Verification items for the finished model (mm, model axes). A direction names the side the tool comes from. Round coordinates to 2 decimals unless told otherwise and drop trailing zeros. Write each loop counter-clockwise with the first axis right and the second up, starting at its lowest first coordinate (ties: lowest second). Pieces come first, ordered by that corner, then holes. Notation, with made-up numbers: M 66,25.25 L 107,25.25 A15 cw 107,46.25 Z; hole C 61.5,22 d1. An arc over 180 degrees is marked long. Use a Markdown table: item, result. Add a question column.
from build123d import *

# Parameters (mm, degrees)
SKETCH_1_W           = 80
SKETCH_1_H           = 24
SKETCH_1_R           = 1.6
EXTRUDE_1_DEPTH      = 3
SKETCH_2_W           = 80
SKETCH_2_H           = 70
EXTRUDE_2_DEPTH      = 4
SKETCH_3_W           = 80
SKETCH_3_H           = 18
EXTRUDE_3_DEPTH      = 4
SKETCH_4_W           = 80
SKETCH_4_H           = 18
CUT_EXTRUDE_1_DEPTH  = 0.6
FILLET_1_R           = 5
FILLET_2_R           = 5
SKETCH_5_W           = 16
SKETCH_5_H           = 67
EXTRUDE_4_DEPTH      = 4
SKETCH_6_W           = 16
SKETCH_6_H           = 40
EXTRUDE_5_DEPTH      = 4
EXTRUDE_6_DEPTH      = 35
EXTRUDE_6_DEPTH_BACK = 35
SKETCH_9_W           = 16
SKETCH_9_H           = 15
EXTRUDE_7_DEPTH      = 4
EXTRUDE_9_DEPTH      = 70


with BuildPart() as part:
    # 草图1 → 凸台-拉伸1 (new body)
    with BuildSketch(Plane.XY):
        Rectangle(SKETCH_1_W, SKETCH_1_H)
        with Locations((-22.5, 0)):
            Circle(SKETCH_1_R, mode=Mode.SUBTRACT)
        with Locations(Location((22.5, 0, 0), (0, 0, 180))):
            Circle(SKETCH_1_R, mode=Mode.SUBTRACT)
    extrude(amount=EXTRUDE_1_DEPTH)

    # 草图2 → 凸台-拉伸2 (add)
    with BuildSketch(Plane.XZ.offset(12)):
        with Locations((0, 35)):
            Rectangle(SKETCH_2_W, SKETCH_2_H)
    extrude(amount=EXTRUDE_2_DEPTH)

    # 草图3 → 凸台-拉伸3 (add)
    with BuildSketch(Plane.XZ.offset(16)):
        with Locations((0, -9)):
            Rectangle(SKETCH_3_W, SKETCH_3_H)
    extrude(amount=-EXTRUDE_3_DEPTH)

    # 草图4 → 切除-拉伸1 (cut)
    with BuildSketch(Plane(origin=(0, -12, 0), x_dir=(1, 0, 0), z_dir=(0, 1, 0))):
        with Locations((0, 9)):
            Rectangle(SKETCH_4_W, SKETCH_4_H)
    extrude(amount=-CUT_EXTRUDE_1_DEPTH, mode=Mode.SUBTRACT)

    # 圆角1
    fillet_1_edges = [part.edges().sort_by_distance(p)[0] for p in [
        (-40, -14.3, -18),
        (40, -14.3, -18),
    ]]
    fillet(fillet_1_edges, radius=FILLET_1_R)

    # 圆角2
    fillet_2_edges = [part.edges().sort_by_distance(p)[0] for p in [
        (-40, 12, 1.5),
        (40, 12, 1.5),
    ]]
    fillet(fillet_2_edges, radius=FILLET_2_R)

    # 草图5 → 凸台-拉伸4 (add)
    with BuildSketch(Plane(origin=(0, -12, 0), x_dir=(1, 0, 0), z_dir=(0, 1, 0))):
        with Locations((0, -36.5)):
            Rectangle(SKETCH_5_W, SKETCH_5_H)
    extrude(amount=EXTRUDE_4_DEPTH)

    # 草图6 → 凸台-拉伸5 (add)
    with BuildSketch(Plane.XY.offset(70)):
        with Locations((0, 12)):
            Rectangle(SKETCH_6_W, SKETCH_6_H)
    extrude(amount=-EXTRUDE_5_DEPTH)

    # 草图8 → 凸台-拉伸6 (add, two sides: drawn at the far end of the back side and taken through both)
    with BuildSketch(Plane.ZY.offset(-EXTRUDE_6_DEPTH_BACK)):
        Polygon((3, 12), (78, 55.301270189), (78, 48.373066959), (3, 5.07179677), align=None)
    extrude(amount=EXTRUDE_6_DEPTH + EXTRUDE_6_DEPTH_BACK)

    # 草图9 → 凸台-拉伸7 (add)
    with BuildSketch(Plane(origin=(0, 0, 66), x_dir=(-1, 0, 0), z_dir=(0, 0, -1))):
        with Locations((0, 39.5)):
            Rectangle(SKETCH_9_W, SKETCH_9_H)
    extrude(amount=-EXTRUDE_7_DEPTH)

    # 草图11 → 凸台-拉伸9 (add)
    with BuildSketch(Plane(origin=(35, 0, 0), x_dir=(0, 0, -1), z_dir=(1, 0, 0))):
        Polygon((-78, 48.373066959), (-81, 50.105117767), (-78, 55.301270189), align=None)
    extrude(amount=-EXTRUDE_9_DEPTH)


solid = part.part
1. Cross-section at C-C on z = 22.5. Enter the section's corners in (x, y), plus the area to 3 significant figures.
2. Access from +Z, -Z, +X, -X, +Y, -Y to the whole of each face (thin tool, end or side, straight path). Record for faces 1 (the flat face through (0, 17, 66)), 2 (the flat face through (-1, -12.6, -9)), 3 (the flat face through (-24, -12, 37)), 4 (the flat face through (8, -9, 51)), 5 (the cylindrical face through (38, 11, 2)).
3. Release check for a two-part mould opening along Z. For faces 6 (the flat face through (0, -8, 34)), 7 (the flat face through (0.49, 33.35, 39.98)), 8 (the flat face through (0, 12, 1)) record: +Z half, -Z half, draft (parallel to the pull), parting line (faces both ways), or undercut.
4. Cross-section at A-A on y = 0. Enter the section's corners in (x, z).
5. Cross-section at B-B on x = -22.5. Enter the section's corners in (y, z).
6. Cross-section at D-D on y = 39. Enter the section's corners in (x, z), plus the area to 3 significant figures.
7. Scan lines: line 1 along Y through (x, z) = (22.5, 1.45); line 2 along Y through (x, z) = (-2.5, 1); line 3 along Y through (x, z) = (4.5, -9.5). Record each from-to range of solid material in increasing order. Write a range as from..to.
8. Depth check by flat-ended pin: pin 1 Ø17.5 at (x, y) = (-2, 13.5) entering from -Z; pin 2 Ø3 at (x, y) = (-22.5, 0) entering from +Z; pin 3 Ø5 at (x, z) = (17, 3) entering from +Y; pin 4 Ø8 at (x, z) = (3, 20) entering from +Y. Enter the tip coordinate at first touch or a pass-through.
Answer:
| question | item | result |
|---|---|---|
| 1 | outline | M -40,-16 L 40,-16 L 40,-12 L 8,-12 L 8,-8 L -8,-8 L -8,-12 L -40,-12 Z; M -35,16.33 L 35,16.33 L 35,23.26 L -35,23.26 Z |
| 1 | area | 869 mm^2 |
| 2 | face 1 | +X, -X |
| 2 | face 2 | -Z, +X, -X, +Y |
| 2 | face 3 | +Z, -X |
| 2 | face 4 | +Z, +X |
| 2 | face 5 | +Z, -Z, +X, +Y |
| 3 | face 6 | undercut |
| 3 | face 7 | -Z half |
| 3 | face 8 | draft |
| 4 | outline | M -40,0 L -24.1,0 L -24.1,3 L -40,3 Z; M -20.9,0 L 20.9,0 L 20.9,3 L -20.9,3 Z; M -8,66 L 8,66 L 8,70 L -8,70 Z; M 24.1,0 L 40,0 L 40,3 L 24.1,3 Z |
| 5 | outline | M -16,-18 L -12.6,-18 L -12.6,0 L -1.6,0 L -1.6,3 L -12,3 L -12,70 L -16,70 Z; M 1.6,0 L 12,0 L 12,3 L 55.3,78 L 50.11,81 L 5.07,3 L 1.6,3 Z |
| 6 | outline | M -35,49.77 L 35,49.77 L 35,61.77 L -35,61.77 Z; M -8,66 L 8,66 L 8,70 L -8,70 Z |
| 6 | area | 904 mm^2 |
| 7 | line 1 | y = -16..-1.6, 1.6..12 |
| 7 | line 2 | y = -16..12 |
| 7 | line 3 | y = -16..-12.6 |
| 8 | pin 1 | stops at z = 0 |
| 8 | pin 2 | passes through |
| 8 | pin 3 | stops at y = 13.44 |
| 8 | pin 4 | stops at y = 24.12 |
